from build123d import *

# Parameters (mm, degrees)
F1_DEPTH = 25.4
F3_DEPTH = 25.4
F4_SIZE  = 2.54


with BuildPart() as f1:
    # F0 (on Top) → F1 (new body)
    with BuildSketch(Plane.XY):
        with BuildLine():
            ThreePointArc((0, -95.25), (-23.5464301965, -105.7014525143), (-31.5908511281, -130.175))
            ThreePointArc((-31.5908511281, -130.175), (0, -158.75), (31.5908511281, -130.175))
            ThreePointArc((31.5908511281, -130.175), (31.7101878213, -128.5894931081), (31.75, -127))
            ThreePointArc((31.75, -127), (22.4506403027, -104.5493596973), (0, -95.25))
        make_face()
        with BuildLine():
            ThreePointArc((25.4, -127), (-17.9605122421, -144.9605122421), (0, -101.6))
            ThreePointArc((0, -101.6), (17.9605122421, -109.0394877579), (25.4, -127))
        make_face(mode=Mode.SUBTRACT)
        with BuildLine():
            Line((31.5908511281, -130.175), (38.0502351456, -65.9049405121))
            Line((38.0502351456, -65.9049405121), (0, -48.7559073592))
            Line((0, -48.7559073592), (0, -95.25))
            ThreePointArc((0, -95.25), (22.4506403027, -104.5493596973), (31.75, -127))
            ThreePointArc((31.75, -127), (31.7101878213, -128.5894931081), (31.5908511281, -130.175))
        make_face()
        with BuildLine():
            ThreePointArc((-18.2641128699, -40.5243714458), (-36.0793714458, -25.9630787095), (-44.2271915794, -4.445))
            Line((-44.2271915794, -4.445), (-31.5908511281, -130.175))
            ThreePointArc((-31.5908511281, -130.175), (-23.5464301965, -105.7014525143), (0, -95.25))
            Line((0, -95.25), (0, -48.7559073592))
            Line((0, -48.7559073592), (-18.2641128699, -40.5243714458))
        make_face()
        with BuildLine():
            Line((42.2238543576, -24.3779536796), (38.4948291982, -22.225))
            ThreePointArc((38.4948291982, -22.225), (22.225, -38.4948291982), (0, -44.45))
            Line((0, -44.45), (0, -48.7559073592))
            Line((0, -48.7559073592), (38.0502351456, -65.9049405121))
            Line((38.0502351456, -65.9049405121), (42.2238543576, -24.3779536796))
        make_face()
        with BuildLine():
            ThreePointArc((0, -44.45), (-9.3406153233, -43.4575126461), (-18.2641128699, -40.5243714458))
            Line((-18.2641128699, -40.5243714458), (0, -48.7559073592))
            Line((0, -48.7559073592), (0, -44.45))
        make_face()
        with BuildLine():
            ThreePointArc((0, -44.45), (22.225, -38.4948291982), (38.4948291982, -22.225))
            Line((38.4948291982, -22.225), (21.9970452561, -12.7))
            ThreePointArc((21.9970452561, -12.7), (12.7, -21.9970452561), (0, -25.4))
            Line((0, -25.4), (0, -44.45))
        make_face()
        with BuildLine():
            ThreePointArc((44.2271915794, -4.445), (44.3942629498, -2.2252903514), (44.45, 0))
            ThreePointArc((44.45, 0), (39.5592046725, 20.2699734998), (25.9630787095, 36.0793714458))
            ThreePointArc((25.9630787095, 36.0793714458), (-22.225, 38.4948291982), (-44.2271915794, -4.445))
            ThreePointArc((-44.2271915794, -4.445), (-36.0793714458, -25.9630787095), (-18.2641128699, -40.5243714458))
            ThreePointArc((-18.2641128699, -40.5243714458), (-9.3406153233, -43.4575126461), (0, -44.45))
            Line((0, -44.45), (0, -25.4))
            ThreePointArc((0, -25.4), (-17.9605122421, 17.9605122421), (25.4, 0))
            ThreePointArc((25.4, 0), (24.5345159877, -6.5740037456), (21.9970452561, -12.7))
            Line((21.9970452561, -12.7), (38.4948291982, -22.225))
            ThreePointArc((38.4948291982, -22.225), (42.3056175984, -13.6395461661), (44.2271915794, -4.445))
        make_face()
        with BuildLine():
            Line((42.2238543576, -24.3779536796), (44.2271915794, -4.445))
            ThreePointArc((44.2271915794, -4.445), (42.3056175984, -13.6395461661), (38.4948291982, -22.225))
            Line((38.4948291982, -22.225), (42.2238543576, -24.3779536796))
        make_face()
        with BuildLine():
            Line((82.4889197105, -47.625), (42.2238543576, -24.3779536796))
            Line((42.2238543576, -24.3779536796), (38.0502351456, -65.9049405121))
            Line((38.0502351456, -65.9049405121), (96.9394313736, -92.4459796041))
            ThreePointArc((96.9394313736, -92.4459796041), (79.766927996, -73.2425329758), (82.4889197105, -47.625))
        make_face()
        with BuildLine():
            ThreePointArc((25.9630787095, 36.0793714458), (39.5592046725, 20.2699734998), (44.45, 0))
            ThreePointArc((44.45, 0), (44.3942629498, -2.2252903514), (44.2271915794, -4.445))
            Line((44.2271915794, -4.445), (42.2238543576, -24.3779536796))
            Line((42.2238543576, -24.3779536796), (82.4889197105, -47.625))
            ThreePointArc((82.4889197105, -47.625), (103.3133581926, -32.4589195385), (128.5302825017, -37.7290203959))
            Line((128.5302825017, -37.7290203959), (25.9630787095, 36.0793714458))
        make_face()
        with BuildLine():
            ThreePointArc((141.7352262806, -63.5), (138.2418010467, -49.0214475002), (128.5302825017, -37.7290203959))
            ThreePointArc((128.5302825017, -37.7290203959), (103.3133581926, -32.4589195385), (82.4889197105, -47.625))
            ThreePointArc((82.4889197105, -47.625), (79.766927996, -73.2425329758), (96.9394313736, -92.4459796041))
            ThreePointArc((96.9394313736, -92.4459796041), (127.216861602, -90.1670816579), (141.7352262806, -63.5))
        make_face()
        with BuildLine():
            ThreePointArc((135.3852262806, -63.5), (103.411222535, -88.0345159877), (87.9881810245, -50.8))
            ThreePointArc((87.9881810245, -50.8), (116.5592300262, -38.9654840123), (135.3852262806, -63.5))
        make_face(mode=Mode.SUBTRACT)
    extrude(amount=F1_DEPTH)

    # F2 (on face) → F3 (cut)
    with BuildSketch(Plane(origin=(0, 0, 0), x_dir=(1, 0, 0), z_dir=(0, 0, -1))):
        with BuildLine():
            ThreePointArc((32.1448291982, 33.2235226281), (27.4963065702, 15.875), (44.8448291982, 11.2264773719))
            Line((44.8448291982, 11.2264773719), (66.8418744543, 23.9264773719))
            ThreePointArc((66.8418744543, 23.9264773719), (71.4903970824, 41.275), (54.1418744543, 45.9235226281))
            Line((54.1418744543, 45.9235226281), (32.1448291982, 33.2235226281))
        make_face()
        with BuildLine():
            ThreePointArc((-12.7, 44.45), (0, 31.75), (12.7, 44.45))
            Line((12.7, 44.45), (12.7, 69.85))
            ThreePointArc((12.7, 69.85), (0, 82.55), (-12.7, 69.85))
            Line((-12.7, 69.85), (-12.7, 44.45))
        make_face()
    extrude(amount=-F3_DEPTH, mode=Mode.SUBTRACT)

    # F4
    f4_edges = [f1.edges().sort_by_distance(p)[0] for p in [
        (43.143352, -39.573523, 25.4),
        (131.982272, -76.2, 25.4),
        (-12.7, -57.15, 25.4),
        (-25.4, -127, 25.4),
        (0, 25.4, 25.4),
        (27.496307, -15.875, 0),
        (131.982272, -76.2, 0),
        (0, 25.4, 0),
        (12.7, -57.15, 0),
        (-25.4, -127, 0),
    ]]
    chamfer(f4_edges, length=F4_SIZE)


solid = f1.part
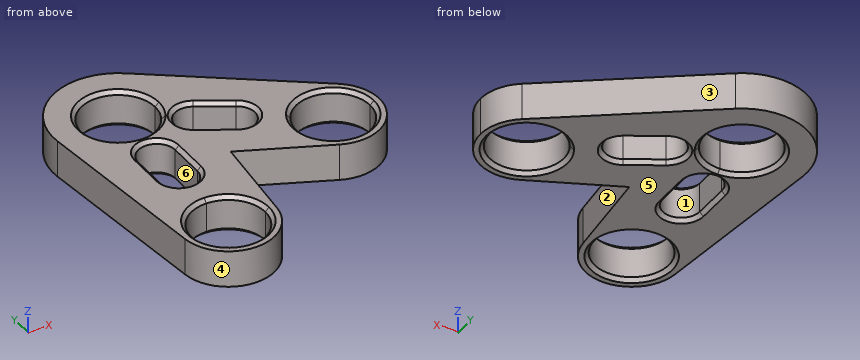
Verification items for the finished model (mm, model axes). Face numbers are marked on the shaded views. A direction names the side the tool comes from. Coordinates: 2 decimals unless noted, no trailing zeros. Write each loop counter-clockwise with the first axis right and the second up, starting at its lowest first coordinate (ties: lowest second). Pieces come first, ordered by that corner, then holes. Notation, with made-up numbers: (49.25, -17) - (72.25, -17) arc R10 ccw to (72.25, -8) - close; hole circle Ø8 at (8.5, 62.25). An arc over 180 degrees is marked (long way). Answer as a JSON object with one key per item and string values.
(1) Cross-section at A-A on z = 6. Record the cut outline in (x, y) (3 decimals), plus the area to 3 significant figures.
Report:
{"outline": "(-44.227, -4.445) - (-31.591, -130.175) arc R31.75 ccw to (31.591, -130.175) - (38.05, -65.905) - (96.939, -92.446) arc R31.75 ccw to (128.53, -37.729) - (25.963, 36.079) arc R44.45 ccw to start; hole circle Ø50.8 at (0, -127); hole circle Ø50.8 at (0, 0); hole (-12.7, -69.85) arc R12.7 ccw to (12.7, -69.85) - (12.7, -44.45) arc R12.7 ccw to (-12.7, -44.45) - close; hole (32.145, -33.224) - (54.142, -45.924) arc R12.7 ccw to (66.842, -23.926) - (44.845, -11.226) arc R12.7 ccw to start; hole circle Ø50.8 at (109.985, -63.5)", "area": "13,400 mm^2"}
(2) Cross-section at B-B on y = -80. Give the number of separate pieces and of enclosed holes in the cut face, plus the area to 3 significant figures.
Report:
{"separate pieces": "4", "enclosed holes": "0", "area": "2,180 mm^2"}
(3) Gauge pin test, flat ends, axial feed: pin 1 Ø8 at (x, y) = (5.5, 20.5) entering from -Z; pin 2 Ø6 at (y, z) = (-59, 9.5) entering from -X; pin 3 Ø1 at (x, z) = (46.5, 19) entering from +Y; pin 4 Ø1 at (x, z) = (75.5, 3) entering from +Y. Record the tip position at first contact, or that the pin passes through.
Report:
{"pin 1": "through", "pin 2": "x = -39.05", "pin 3": "y = 21.66", "pin 4": "y = 0.79"}
(4) Mould release check, pull along X, two halves, no side actions. Record for the marked faces 4, 5 and 6: pulls with the +X half, pulls with the -X half, needs draft (parallel to the pull), parting line crosses it, or undercut.
Report:
{"face 4": "parting line crosses it", "face 5": "needs draft", "face 6": "undercut"}
(5) Thickness scan on line 1 along Y through (x, z) = (0, 16.75); line 2 along Y through (x, z) = (-13.5, 6.5); line 3 along X through (y, z) = (-54, 19.5). Record the ranges inside material, lowest first.
Report:
{"line 1": "-158.75 to -152.4, -101.6 to -82.55, -31.75 to -25.4, 25.4 to 44.45", "line 2": "-155.74 to -148.52, -105.48 to -21.52, 21.52 to 42.35", "line 3": "-39.25 to -12.7, 12.7 to 86.43, 133.54 to 140.28"}
(6) Tool access check on the marked faces 1, 2 and 3. Record the directions out of +Z, -Z, +X, -X, +Y, -Y that give a thin tool (end or side, any length) a straight path to the whole face; none if there is none.
Report:
{"face 1": "+Z, -Z", "face 2": "+Z, -Z, -Y", "face 3": "+Z, -Z, +X, +Y"}
